Part model, mm, in its own coordinate system. Give positions to 0.01 mm unless a question says otherwise; leave off trailing zeros. Order: outer loops, then holes, each group sorted by start corner. A loop starts at its lowest first (then second) coordinate and runs counter-clockwise, first axis right, second up. Notation, with made-up numbers: (-36, 52) - (7, 52) arc R26 cw to (7, 75) - close; hole circle Ø10 at (49, 55.25). An arc over 180 degrees is marked (long way). Use one line per item in the form item = value. Start each with the question number.
1. Drill centre lines: line 1 (X direction, y = -5.75, z = 270); line 2 (X direction, y = -13.75, z = 74); line 3 (X direction, y = -20.75, z = 183). Where is each one in solid material? Low to high.
2. Pin check, flat tips, straight feed: P1, Ø14.5, axis at x = -99.9, z = 86.86, coming from the +Y side; P2, Ø20.5, axis at x = -204.9, z = 268.74, coming from the +Y side. Stop position of each tip, or through.
3. Band-saw the part on A-A, the plane z = 177.8. List the corners of the cut face in (x, y).
4. Band-saw the part on B-B, the plane y = -15.75. State how many separate pieces and enclosed holes the cut face has, plus the area to 3 significant figures.
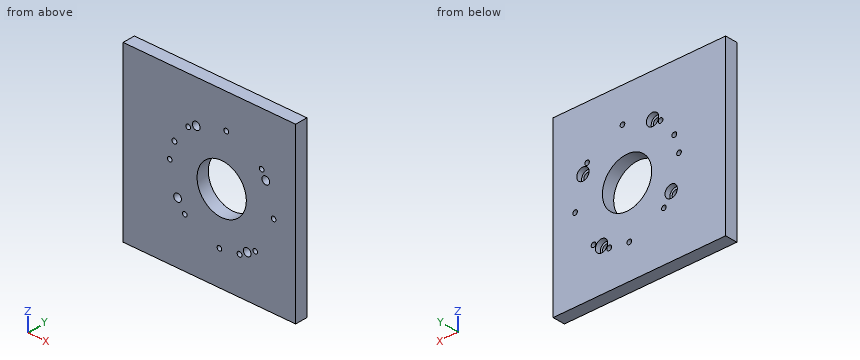
from build123d import *

# Parameters (mm, degrees)
F0_W     = 355.6
F0_H     = 355.6
F1_DEPTH = 25.4
F2_R     = 4.7625
F2_R_2   = 4.9784
F2_R_3   = 50.8
F3_DEPTH = 25.401
F4_R     = 7.9375
F5_DEPTH = 25.401
F6_R     = 12.7
F7_DEPTH = 10.922


with BuildPart() as f1:
    # F0 (on Front) → F1 (new body)
    with BuildSketch(Plane.XZ):
        with Locations((-177.8, 177.8)):
            Rectangle(F0_W, F0_H)
    extrude(amount=F1_DEPTH)

    # F2 (on face) → F3 (cut, through all)
    with BuildSketch(Plane.XZ.offset(25.4)):
        with Locations((-259.49093, 187.169242)):
            Circle(F2_R)
        with Locations((-221.499668, 260.149778)):
            Circle(F2_R)
        with Locations((-143.030758, 284.89093)):
            Circle(F2_R)
        with Locations((-70.050222, 246.899668)):
            Circle(F2_R)
        with Locations((-45.30907, 168.430758)):
            Circle(F2_R)
        with Locations((-83.300332, 95.450222)):
            Circle(F2_R)
        with Locations((-157.089084, 70.402316)):
            Circle(F2_R)
        with Locations((-228.413979, 101.786021)):
            Circle(F2_R)
        with Locations((-249.828087, 223.231463)):
            Circle(F2_R_2)
        with Locations((-115.632835, 76.783043)):
            Circle(F2_R_2)
        with Locations((-152.4, 177.8)):
            Circle(F2_R_3)
    extrude(amount=-F3_DEPTH, mode=Mode.SUBTRACT)

    # F4 (on face) → F5 (cut, through all)
    with BuildSketch(Plane.XZ.offset(25.4)):
        with Locations((-204.9018, 268.735785)):
            Circle(F4_R)
        with Locations((-243.335785, 125.2982)):
            Circle(F4_R)
        with Locations((-99.8982, 86.864215)):
            Circle(F4_R)
        with Locations((-61.464215, 230.3018)):
            Circle(F4_R)
    extrude(amount=-F5_DEPTH, mode=Mode.SUBTRACT)

    # F6 (on face) → F7 (cut)
    with BuildSketch(Plane(origin=(0, 0, 0), x_dir=(-1, 0, 0), z_dir=(0, 1, 0))):
        with Locations((204.9018, 268.735785)):
            Circle(F6_R)
        with Locations((243.335785, 125.2982)):
            Circle(F6_R)
        with Locations((99.8982, 86.864215)):
            Circle(F6_R)
        with Locations((61.464215, 230.3018)):
            Circle(F6_R)
    extrude(amount=-F7_DEPTH, mode=Mode.SUBTRACT)


solid = f1.part
From the geometry:
q1.line_1 = -355.6 to -217.54, -192.26 to 0
q1.line_2 = -355.6 to -160.21, -153.97 to -119.76, -111.5 to 0
q1.line_3 = -355.6 to -261.79, -257.19 to -202.93, -101.87 to 0
q2.P1 = through
q2.P2 = -10.92
q3.outline = (-355.6, -25.4) - (-203.2, -25.4) - (-203.2, 0) - (-355.6, 0) - close; (-101.6, -25.4) - (0, -25.4) - (0, 0) - (-101.6, 0) - close
q4.separate_pieces = 1
q4.enclosed_holes = 15
q4.area = 117,000 mm²
